Here's how the part is built. I have some questions about the finished solid (model axes, mm). A direction names the side the tool comes from. Round coordinates to 2 decimals unless told otherwise and drop trailing zeros. Write each loop counter-clockwise with the first axis right and the second up, starting at its lowest first coordinate (ties: lowest second). Pieces come first, ordered by that corner, then holes. Notation, with made-up numbers: (83.25, 74) -> (111.25, 74) arc R24 ccw to (111.25, 85) -> close; hole circle Ø4 at (34, 58.25). An arc over 180 degrees is marked (long way). Put each result on its own line as item: value. Start each with the question number.
1. Which directions (+Z, -Z, +X, -X, +Y, -Y) give clear straight access to the entire face, cutting with the end or side of a thin tool? Please do faces 4 (the face through (164, 101.6, -153)), 5 (the face through (330.2, 50, -77)).
2. I need wall thicknesses on probe 1 along X at (y, z) = (73.5, -115) (3 decimals); probe 2 along X at (y, z) = (76, -154) (3 decimals); probe 3 along Y at (x, z) = (165, -154). Which ranges of each line are inside material? Lowest first, please. Write a range as from..to.
3. Suppose I cut it at C-C (y = 76.2). Please give me the cut outline in (x, z) (3 decimals), then the cut area to 3 significant figures.
4. Suppose I cut it at A-A (x = 165.1). Please give me the cut outline in (y, z) (3 decimals).
5. For pin 1 (7.5 mm diameter, centred on x = 165.1, y = 76.2, fed in from +Z), with a flat end and sliding along its axis, tell me the tip position at first contact or that it passes through.
6. We'd pull the mould along X, two halves only. Please class faces 1 (the face through (0, 50, -75)), 2 (the face through (-3.175, 50, -79)), 3 (the face through (167, 50, -155.575)): +X half, -X half, draft (parallel to the pull), parting line (faces both ways), or undercut.
7. Suppose I cut it at B-B (z = -127). Please give me the cut outline in (x, y) (3 decimals).
8. Suppose I cut it at D-D (x = 307). Please give me the cut outline in (y, z) (3 decimals).
```python
from build123d import *

# Parameters (mm, degrees)
BOSS_EXTRUDE1_DEPTH = 101.6
CUT_EXTRUDE1_REACH  = 157.575
SKETCH2_R           = 6.35


with BuildPart() as part:
    # Sketch1 → Boss-Extrude1 (new body)
    with BuildSketch(Plane(origin=(0, 0, 0), x_dir=(1, 0, 0), z_dir=(0, 1, 0))):
        Polygon((0, 0), (0, 152.4), (330.2, 152.4), (330.2, 0), (333.375, 0), (333.375, 155.575), (-3.175, 155.575), (-3.175, 0), align=None)
    extrude(amount=BOSS_EXTRUDE1_DEPTH)

    # Sketch2 → Cut-Extrude1 (cut, up to next)
    with BuildSketch(Plane(origin=(0, 0, -155.575), x_dir=(-1, 0, 0), z_dir=(0, 0, -1)), mode=Mode.PRIVATE) as cut_extrude1_sk1:
        with Locations((-165.1, 76.2)):
            Circle(SKETCH2_R)
    cut_extrude1_tool1 = extrude(cut_extrude1_sk1.sketch, amount=-CUT_EXTRUDE1_REACH, mode=Mode.PRIVATE) & part.part
    add(cut_extrude1_tool1.solids().sort_by_distance((165.1, 76.2, -155.575))[0], mode=Mode.SUBTRACT)


solid = part.part
```
Verdict:
1. face 4: +Z, -Z, +X, -X, +Y
1. face 5: +Z, +Y, -Y
2. probe 1: x = -3.175..0, 330.2..333.375
2. probe 2: x = -3.175..158.753, 171.447..333.375
2. probe 3: y = 0..69.85, 82.55..101.6
3. outline: (-3.175, -155.575) -> (158.75, -155.575) -> (158.75, -152.4) -> (0, -152.4) -> (0, 0) -> (-3.175, 0) -> close; (171.45, -155.575) -> (333.375, -155.575) -> (333.375, 0) -> (330.2, 0) -> (330.2, -152.4) -> (171.45, -152.4) -> close
3. area: 2,000 mm^2
4. outline: (0, -155.575) -> (69.85, -155.575) -> (69.85, -152.4) -> (0, -152.4) -> close; (82.55, -155.575) -> (101.6, -155.575) -> (101.6, -152.4) -> (82.55, -152.4) -> close
5. pin 1: passes through
6. face 1: undercut
6. face 2: -X half
6. face 3: draft
7. outline: (-3.175, 0) -> (0, 0) -> (0, 101.6) -> (-3.175, 101.6) -> close; (330.2, 0) -> (333.375, 0) -> (333.375, 101.6) -> (330.2, 101.6) -> close
8. outline: (0, -155.575) -> (101.6, -155.575) -> (101.6, -152.4) -> (0, -152.4) -> close
